```python
from build123d import *

# Parameters (mm, degrees)
F1_DEPTH = 3
F2_R     = 3
F3_R     = 2
F5_DEPTH = 0.5
F6_R     = 0.5


with BuildPart() as f1:
    # F0 (on Top) → F1 (new body, symmetric)
    with BuildSketch(Plane.XY):
        with BuildLine():
            Line((-15.1986841536, -5), (15.1986841536, -5))
            ThreePointArc((15.1986841536, -5), (16, 0), (15.1986841536, 5))
            Line((15.1986841536, 5), (-15.1986841536, 5))
            ThreePointArc((-15.1986841536, 5), (-16, 0), (-15.1986841536, -5))
        make_face()
        with BuildLine():
            ThreePointArc((13.6747943312, 3), (14, 0), (13.6747943312, -3))
            Line((13.6747943312, -3), (-13.6747943312, -3))
            ThreePointArc((-13.6747943312, -3), (-14, 0), (-13.6747943312, 3))
            Line((-13.6747943312, 3), (13.6747943312, 3))
        make_face(mode=Mode.SUBTRACT)
    extrude(amount=F1_DEPTH, both=True)

    # F2
    f2_edges = [f1.edges().sort_by_distance(p)[0] for p in [
        (-15.198684, 5, 0),
        (15.198684, 5, 0),
        (15.198684, -5, 0),
        (-15.198684, -5, 0),
    ]]
    fillet(f2_edges, radius=F2_R)

    # F3
    f3_edges = [f1.edges().sort_by_distance(p)[0] for p in [
        (13.674794, 3, 0),
        (13.674794, -3, 0),
        (-13.674794, -3, 0),
        (-13.674794, 3, 0),
    ]]
    fillet(f3_edges, radius=F3_R)

    # F4 (on Top) → F5 (join, symmetric)
    with BuildSketch(Plane.XY):
        Polygon((-4, 3), (-8.3, 3), (-8.15, 2), (-4.15, 2), align=None)
        Polygon((8.3, 3), (4, 3), (4.15, 2), (8.15, 2), align=None)
    extrude(amount=F5_DEPTH, both=True)

    # F6
    f6_edges = [f1.edges().sort_by_distance(p)[0] for p in [
        (0, -5, 3),
        (14.796563, -4.278664, 3),
        (16, 0, 3),
        (14.796563, 4.278664, 3),
        (0, 5, 3),
        (-14.796563, -4.278664, 3),
        (-16, 0, 3),
        (-14.796563, 4.278664, 3),
        (-16, 0, -3),
        (-14.796563, 4.278664, -3),
        (-14.796563, -4.278664, -3),
        (0, -5, -3),
        (0, 5, -3),
        (14.796563, -4.278664, -3),
        (16, 0, -3),
        (14.796563, 4.278664, -3),
    ]]
    fillet(f6_edges, radius=F6_R)


solid = f1.part
```
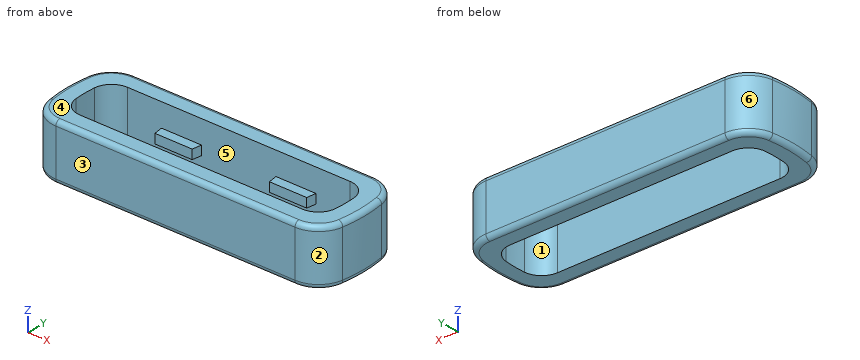
Here's how the part is built. I have some questions about the finished solid (model axes, mm). Face numbers are marked on the shaded views. A direction names the side the tool comes from. Coordinates: 2 decimals unless noted, no trailing zeros. Order: outer loops, then holes, each group sorted by start corner. A loop starts at its lowest first (then second) coordinate and runs counter-clockwise, first axis right, second up.
1) Imagine slicing it at D-D on z = 1.8. List the corners of the cut face in (x, y) for me.
2) Imagine slicing it at C-C on x = -6.5. List the corners of the cut face in (y, z) for me.
3) We'd pull the mould along Y, two halves only. Please class the marked faces 3, 4, 5 and 6: +Y half, -Y half, draft (parallel to the pull), parting line (faces both ways), or undercut.
4) Imagine slicing it at B-B on z = 0.15. List the corners of the cut face in (x, y) for me, and give its area (3 significant figures).
5) Which directions (+Z, -Z, +X, -X, +Y, -Y) give clear straight access to the entire face, cutting with the end or side of a thin tool? Please do the marked faces 1 and 2.
6) Imagine slicing it at A-A on x = 11.5. List the corners of the cut face in (y, z) for me, and give its area (3 significant figures).
7) Will these pins go through, and if not, where does the flat tip stop? pin 1 (1.5 mm diameter, centred on y = -1.5, z = 1, fed in from +X); pin 2 (0.5 mm diameter, centred on x = 6.5, y = 2.5, fed in from -Z); pin 3 (5 mm diameter, centred on x = -8.5, y = 0, fed in from +Z).
8) I need wall thicknesses on line 1 (Y direction, x = 2, z = -1.85); line 2 (Y direction, x = 13.5, z = -1); line 3 (X direction, y = 2, z = 1.9). Which ranges of each line are inside material? Lowest first, please.
Response values:
1. outline: (-15.81, -2.46) arc R3 ccw to (-12.85, -5) - (12.85, -5) arc R3 ccw to (15.81, -2.46) arc R16 ccw to (15.81, 2.46) arc R3 ccw to (12.85, 5) - (-12.85, 5) arc R3 ccw to (-15.81, 2.46) arc R16 ccw to start; hole (-13.95, -1.17) arc R2 ccw to (-11.96, -3) - (11.96, -3) arc R2 ccw to (13.95, -1.17) arc R14 ccw to (13.95, 1.17) arc R2 ccw to (11.96, 3) - (-11.96, 3) arc R2 ccw to (-13.95, 1.17) arc R14 ccw to start
2. outline: (-5, -2.5) arc R0.5 ccw to (-4.5, -3) - (-3, -3) - (-3, 3) - (-4.5, 3) arc R0.5 ccw to (-5, 2.5) - close; (2, -0.5) - (3, -0.5) - (3, -3) - (4.5, -3) arc R0.5 ccw to (5, -2.5) - (5, 2.5) arc R0.5 ccw to (4.5, 3) - (3, 3) - (3, 0.5) - (2, 0.5) - close
3. face 3: -Y half
3. face 4: draft
3. face 5: undercut
3. face 6: +Y half
4. outline: (-15.81, -2.46) arc R3 ccw to (-12.85, -5) - (12.85, -5) arc R3 ccw to (15.81, -2.46) arc R16 ccw to (15.81, 2.46) arc R3 ccw to (12.85, 5) - (-12.85, 5) arc R3 ccw to (-15.81, 2.46) arc R16 ccw to start; hole (-13.95, -1.17) arc R2 ccw to (-11.96, -3) - (11.96, -3) arc R2 ccw to (13.95, -1.17) arc R14 ccw to (13.95, 1.17) arc R2 ccw to (11.96, 3) - (8.3, 3) - (8.15, 2) - (4.15, 2) - (4, 3) - (-4, 3) - (-4.15, 2) - (-8.15, 2) - (-8.3, 3) - (-11.96, 3) arc R2 ccw to (-13.95, 1.17) arc R14 ccw to start
4. area: 154 mm2
5. face 1: +Z, -Z
5. face 2: +Z, -Z, +X, -Y
6. outline: (-5, -2.5) arc R0.5 ccw to (-4.5, -3) - (-3, -3) - (-3, 3) - (-4.5, 3) arc R0.5 ccw to (-5, 2.5) - close; (3, -3) - (4.5, -3) arc R0.5 ccw to (5, -2.5) - (5, 2.5) arc R0.5 ccw to (4.5, 3) - (3, 3) - close
6. area: 23.8 mm2
7. pin 1: stops at x = 15.98
7. pin 2: stops at z = -0.5
7. pin 3: stops at z = 0.5
8. line 1: y = -5 to -3, 3 to 5
8. line 2: y = -4.93 to -2.27, 2.27 to 4.93
8. line 3: x = -15.87 to -13.69, 13.69 to 15.87
